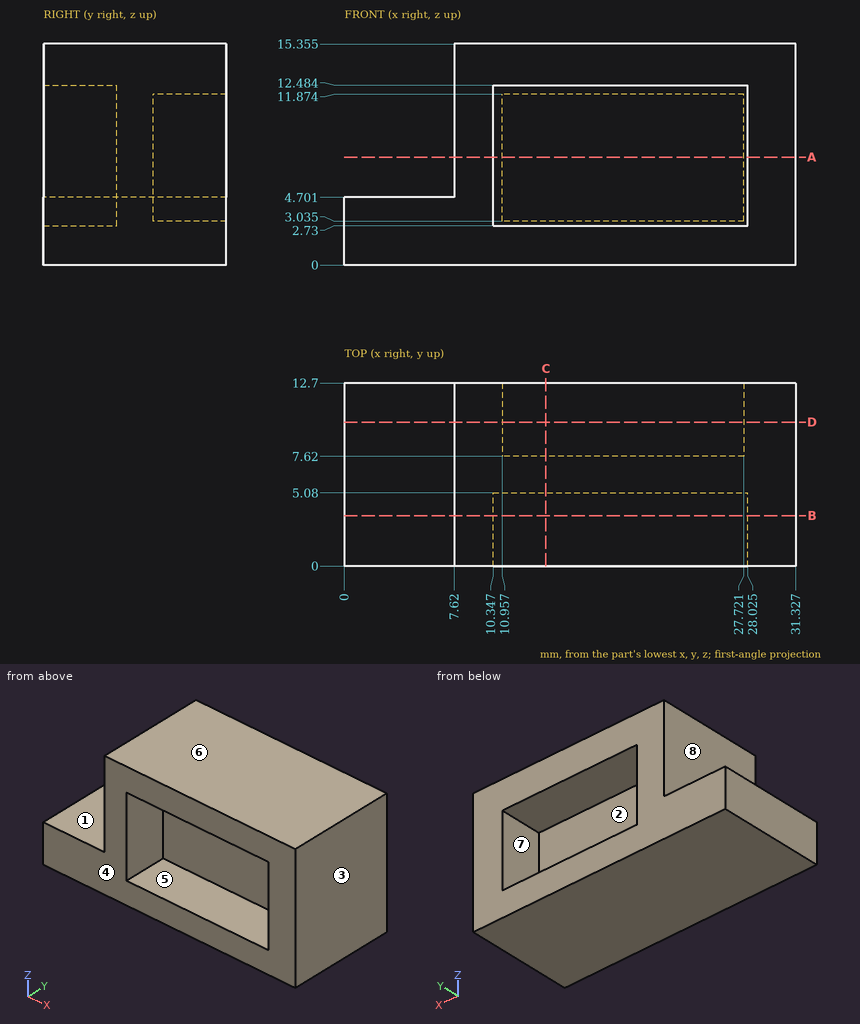
Part print with two shaded views. Sizes in mm from the minimum x, y, z corner. A direction names the side the tool comes from. Coordinates: 2 decimals unless noted, no trailing zeros. Write each loop counter-clockwise with the first axis right and the second up, starting at its lowest first coordinate (ties: lowest second). Pieces come first, ordered by that corner, then holes. Notation, with made-up numbers: (3.5, 36) -> (50.5, 36) arc R6 ccw to (50.5, 46) -> close; hole circle Ø5 at (43, 22). An arc over 180 degrees is marked (long way). Return JSON: item names as keys, results as strings. Group by question number.
Q1. Which spindle directions (+Z, -Z, +X, -X, +Y, -Y) get a long thin tool onto all of the face, cutting with end or side? Do the marked faces 1, 2, 3, 4 and 5. Say none if no direction does.
Q2. Drill centre lines: line 1 (X direction, y = 9, z = 4.5); line 2 (Z direction, x = 14.5, y = 1.5) (1 decimal); line 3 (X direction, y = 10.75, z = 8.5). Where is each one in solid material? Low to high.
Q3. Cut at D-D, the plane y = 10. Give the cut face in (x, z) (1 decimal).
Q4. Cut at A-A, the plane z = 7.5. Give the cut face in (x, y) (1 decimal), then the cut area to 3 significant figures.
Q5. Cut at B-B, the plane y = 3.5. Give the cut face in (x, z) (1 decimal).
Q6. Pull direction X, two halves, no side cores. Call the marked faces 6, 7 and 8: released by +X, released by -X, zero draft, split by the parting line, or undercut.
Q7. Flat gauge pins, fed straight in: pin 1 (5.5 mm diameter, centred on y = 3, z = 8.5, fed in from -X); pin 2 (2.5 mm diameter, centred on x = 17.5, y = 1.5, fed in from -Z); pin 3 (4 mm diameter, centred on x = 3.5, y = 6, fed in from +Z); pin 4 (7 mm diameter, centred on x = 18, z = 7.5, fed in from +Y). Where does each tip first touch, or does it go through?
Q8. Cut at C-C, the plane x = 14. Give the cut face in (y, z) (1 decimal).
Returned:
{
 "1": {"face 1": "+Z, -X, +Y, -Y", "face 2": "+Y", "face 3": "+Z, -Z, +X, +Y, -Y", "face 4": "+Z, -Z, +X, -X, -Y", "face 5": "-Y"},
 "2": {"line 1": "x = 0 to 10.96, 27.72 to 31.33", "line 2": "z = 0 to 2.7, 12.5 to 15.4", "line 3": "x = 7.62 to 10.96, 27.72 to 31.33"},
 "3": {"outline": "(0, 0) -> (31.3, 0) -> (31.3, 15.4) -> (7.6, 15.4) -> (7.6, 4.7) -> (0, 4.7) -> close; hole (11, 3) -> (27.7, 3) -> (27.7, 11.9) -> (11, 11.9) -> close"},
 "4": {"outline": "(7.6, 0) -> (10.3, 0) -> (10.3, 5.1) -> (28, 5.1) -> (28, 0) -> (31.3, 0) -> (31.3, 12.7) -> (27.7, 12.7) -> (27.7, 7.6) -> (11, 7.6) -> (11, 12.7) -> (7.6, 12.7) -> close", "area": "126 mm2"},
 "5": {"outline": "(0, 0) -> (31.3, 0) -> (31.3, 15.4) -> (7.6, 15.4) -> (7.6, 4.7) -> (0, 4.7) -> close; hole (10.3, 2.7) -> (28, 2.7) -> (28, 12.5) -> (10.3, 12.5) -> close"},
 "6": {"face 6": "zero draft", "face 7": "undercut", "face 8": "released by -X"},
 "7": {"pin 1": "stops at x = 7.62", "pin 2": "stops at z = 0", "pin 3": "stops at z = 4.7", "pin 4": "stops at y = 7.62"},
 "8": {"outline": "(0, 0) -> (12.7, 0) -> (12.7, 3) -> (7.6, 3) -> (7.6, 11.9) -> (12.7, 11.9) -> (12.7, 15.4) -> (0, 15.4) -> (0, 12.5) -> (5.1, 12.5) -> (5.1, 2.7) -> (0, 2.7) -> close"}
}
